The model under review builds one solid part; all positions refer to its coordinate system, in mm. A direction names the side the tool comes from. Round coordinates to 2 decimals unless told otherwise and drop trailing zeros. Write each loop counter-clockwise with the first axis right and the second up, starting at its lowest first coordinate (ties: lowest second). Pieces come first, ordered by that corner, then holes.
Item 1: Clearance check with flat-ended pins moving along their axes: pin 1 Ø10 at (x, z) = (-6.5, 13.5) entering from +Y; pin 2 Ø12 at (x, z) = (41, 70.5) entering from +Y; pin 3 Ø5.5 at (x, z) = (3, 92) entering from -Y; pin 4 Ø1.5 at (x, z) = (16, 33) entering from +Y. State where each tip first meets the part, or that it passes through.
Item 2: Add section A-A (y = -43.5). Give the boundary of the cut face in (x, z), plus the area to 3 significant figures.
Item 3: Machinability: for faces 1 (the face through (-1, 25.492, 41)), 2 (the face through (-24.156, -5, 71)), 3 (the face through (-1, -26.065, 56)), 4 (the face through (44.206, -4, 41)), which of the approach directions +Z, -Z, +X, -X, +Y, -Y give a long, thin tool a straight path to every point of the face, cutting with its end or side? Answer none if there is none.
Item 4: To check wall thickness, follow L1, parallel to Y at x = -29.5, z = 51; L2, parallel to X at y = 16, z = 49; L3, parallel to Z at x = 52, y = -30. State the ranges of each line that lie inside material, in increasing order.
Item 5: Add section B-B (z = 24.5). Give the boundary of the cut face in (x, y), plus the area to 3 significant figures.
Item 6: Add section C-C (z = 55). Give the boundary of the cut face in (x, y), plus the area to 3 significant figures.
```python
from build123d import *

# Parameters (mm, degrees)
F0_W      = 13.366825413
F0_H      = 3.0552744865
F1_DEPTH  = 99.568
F0_W_2    = 19.0954655409
F0_H_2    = 6.1105492059
F2_DEPTH  = 93.726
F0_W_3    = 28.6431992427
F0_H_3    = 11.9346659631
F3_DEPTH  = 88.646
F0_W_4    = 38.3818857372
F0_H_4    = 20.2411934733
F4_DEPTH  = 81.28
F0_W_5    = 49.0753464401
F0_H_5    = 26.9246064126
F5_DEPTH  = 73.914
F0_W_6    = 59.3868978322
F0_H_6    = 35.7085214928
F6_DEPTH  = 67.31
F0_W_7    = 67.9798536003
F0_H_7    = 42.964797467
F7_DEPTH  = 59.182
F0_W_8    = 75.9999491274
F0_H_8    = 49.2663010955
F8_DEPTH  = 52.578
F0_W_9    = 88.7939184904
F0_H_9    = 58.0502152443
F9_DEPTH  = 45.212
F0_W_10   = 100.4421524704
F0_H_10   = 65.4974486679
F10_DEPTH = 36.83
F0_W_11   = 114.7637441754
F0_H_11   = 76.9547224045
F11_DEPTH = 28.194
F0_W_12   = 128.1305700541
F0_H_12   = 86.884368211
F12_DEPTH = 18.288
F0_W_13   = 139.5878568292
F0_H_13   = 98.3416512609
F13_DEPTH = 9.398


# Not quite as in the source:
# - the program builds the solid bodies; features that only make, move or delete a surface that nothing else refers to are left out


with BuildPart() as f1:
    # F0 (on Top) → F1 (new body)
    with BuildSketch(Plane.XY):
        with Locations((1.8140685279, -5.8241172228)):
            Rectangle(F0_W, F0_H)
    extrude(amount=F1_DEPTH)

    # F0 (on Top) → F2 (join)
    with BuildSketch(Plane.XY):
        with Locations((1.0502506047, -5.8241168736)):
            Rectangle(F0_W_2, F0_H_2)
        with Locations((1.8140685279, -5.8241172228)):
            Rectangle(F0_W, F0_H, mode=Mode.SUBTRACT)
    extrude(amount=F2_DEPTH)

    # F0 (on Top) → F3 (join)
    with BuildSketch(Plane.XY):
        with Locations((0.2864324488, -5.9673329815)):
            Rectangle(F0_W_3, F0_H_3)
        with Locations((1.0502506047, -5.8241168736)):
            Rectangle(F0_W_2, F0_H_2, mode=Mode.SUBTRACT)
    extrude(amount=F3_DEPTH)

    # F0 (on Top) → F4 (join)
    with BuildSketch(Plane.XY):
        with Locations((0.1909546554, -5.6331623346)):
            Rectangle(F0_W_4, F0_H_4)
        with Locations((0.2864324488, -5.9673329815)):
            Rectangle(F0_W_3, F0_H_3, mode=Mode.SUBTRACT)
    extrude(amount=F4_DEPTH)

    # F0 (on Top) → F5 (join)
    with BuildSketch(Plane.XY):
        with Locations((0.3819093108, -4.9648210406)):
            Rectangle(F0_W_5, F0_H_5)
        with Locations((0.1909546554, -5.6331623346)):
            Rectangle(F0_W_4, F0_H_4, mode=Mode.SUBTRACT)
    extrude(amount=F5_DEPTH)

    # F0 (on Top) → F6 (join)
    with BuildSketch(Plane.XY):
        with Locations((-0.1909546554, -4.5829112642)):
            Rectangle(F0_W_6, F0_H_6)
        with Locations((0.3819093108, -4.9648210406)):
            Rectangle(F0_W_5, F0_H_5, mode=Mode.SUBTRACT)
    extrude(amount=F6_DEPTH)

    # F0 (on Top) → F7 (join)
    with BuildSketch(Plane.XY):
        with Locations((-0.0954773277, -4.5829117298)):
            Rectangle(F0_W_7, F0_H_7)
        with Locations((-0.1909546554, -4.5829112642)):
            Rectangle(F0_W_6, F0_H_6, mode=Mode.SUBTRACT)
    extrude(amount=F7_DEPTH)

    # F0 (on Top) → F8 (join)
    with BuildSketch(Plane.XY):
        with Locations((-0.0954773277, -4.8693437129)):
            Rectangle(F0_W_8, F0_H_8)
        with Locations((-0.0954773277, -4.5829117298)):
            Rectangle(F0_W_7, F0_H_7, mode=Mode.SUBTRACT)
    extrude(amount=F8_DEPTH)

    # F0 (on Top) → F9 (join)
    with BuildSketch(Plane.XY):
        with Locations((-0.1909546554, -3.5326592624)):
            Rectangle(F0_W_9, F0_H_9)
        with Locations((-0.0954773277, -4.8693437129)):
            Rectangle(F0_W_8, F0_H_8, mode=Mode.SUBTRACT)
    extrude(amount=F9_DEPTH)

    # F0 (on Top) → F10 (join)
    with BuildSketch(Plane.XY):
        with Locations((0.0954773277, -3.8190940395)):
            Rectangle(F0_W_10, F0_H_10)
        with Locations((-0.1909546554, -3.5326592624)):
            Rectangle(F0_W_9, F0_H_9, mode=Mode.SUBTRACT)
    extrude(amount=F10_DEPTH)

    # F0 (on Top) → F11 (join)
    with BuildSketch(Plane.XY):
        with Locations((-0.1909546554, -2.4824105203)):
            Rectangle(F0_W_11, F0_H_11)
        with Locations((0.0954773277, -3.8190940395)):
            Rectangle(F0_W_10, F0_H_10, mode=Mode.SUBTRACT)
    extrude(amount=F11_DEPTH)

    # F0 (on Top) → F12 (join)
    with BuildSketch(Plane.XY):
        with Locations((0.1909509301, -1.718590036)):
            Rectangle(F0_W_12, F0_H_12)
        with Locations((-0.1909546554, -2.4824105203)):
            Rectangle(F0_W_11, F0_H_11, mode=Mode.SUBTRACT)
    extrude(amount=F12_DEPTH)

    # F0 (on Top) → F13 (join)
    with BuildSketch(Plane.XY):
        with Locations((0.1909546554, -1.1457279325)):
            Rectangle(F0_W_13, F0_H_13)
        with Locations((0.1909509301, -1.718590036)):
            Rectangle(F0_W_12, F0_H_12, mode=Mode.SUBTRACT)
    extrude(amount=F13_DEPTH)


solid = f1.part
```
Numbers:
1. pin 1: stops at y = 48.03
1. pin 2: passes through
1. pin 3: stops at y = -8.88
1. pin 4: stops at y = 28.93
2. outline: (-69.6, 0) - (69.98, 0) - (69.98, 9.4) - (64.26, 9.4) - (64.26, 18.29) - (-63.87, 18.29) - (-63.87, 9.4) - (-69.6, 9.4) - close
2. area: 2,450 mm2
3. face 1: +Z, +X, -X, +Y
3. face 2: +Z, -X, +Y, -Y
3. face 3: +Z, +X, -X, -Y
3. face 4: +Z, +X, +Y, -Y
4. L1: y = -29.5 to 19.76
4. L2: x = -38.1 to 37.9
4. L3: z = 0 to 28.19
5. outline: (-57.57, -40.96) - (57.19, -40.96) - (57.19, 35.99) - (-57.57, 35.99) - close
5. area: 8,830 mm2
6. outline: (-34.09, -26.07) - (33.89, -26.07) - (33.89, 16.9) - (-34.09, 16.9) - close
6. area: 2,920 mm2
